```python
from build123d import *

# Parameters (mm, degrees)
SKETCH1_R           = 3.175
SKETCH1_R_2         = 2.286
BOSS_EXTRUDE1_DEPTH = 2.54
SKETCH2_R           = 3.175
BOSS_EXTRUDE2_DEPTH = 3.175


with BuildPart() as part:
    # Sketch1 → Boss-Extrude1 (new body)
    with BuildSketch(Plane(origin=(0, 0, 0), x_dir=(1, 0, 0), z_dir=(0, 1, 0))):
        with BuildLine():
            Line((2.54, 0), (10.16, 0))
            ThreePointArc((10.16, 0), (11.956051224, 0.743948776), (12.7, 2.54))
            Line((12.7, 2.54), (12.7, 25.4))
            ThreePointArc((12.7, 25.4), (6.35, 31.75), (0, 25.4))
            Line((0, 25.4), (0, 2.54))
            ThreePointArc((0, 2.54), (0.743948776, 0.743948776), (2.54, 0))
        make_face()
        with Locations((6.35, 25.4)):
            Circle(SKETCH1_R, mode=Mode.SUBTRACT)
        with Locations((6.35, 6.35)):
            Circle(SKETCH1_R_2, mode=Mode.SUBTRACT)
    extrude(amount=BOSS_EXTRUDE1_DEPTH)

    # Sketch2 → Boss-Extrude2 (add)
    with BuildSketch(Plane(origin=(0, 2.54, 0), x_dir=(1, 0, 0), z_dir=(0, 1, 0))):
        with BuildLine():
            Line((0, 25.4), (0, 16.256))
            Line((0, 16.256), (12.7, 16.256))
            Line((12.7, 16.256), (12.7, 25.4))
            ThreePointArc((12.7, 25.4), (6.35, 31.75), (0, 25.4))
        make_face()
        with Locations((6.35, 25.4)):
            Circle(SKETCH2_R, mode=Mode.SUBTRACT)
    extrude(amount=BOSS_EXTRUDE2_DEPTH)


solid = part.part
```
Could you check a few things on this model? Use its own coordinates, in mm. A direction names the side the tool comes from. Give positions to 0.01 mm unless a question says otherwise; leave off trailing zeros. Write each loop counter-clockwise with the first axis right and the second up, starting at its lowest first coordinate (ties: lowest second). Pieces come first, ordered by that corner, then holes. Notation, with made-up numbers: (48.25, 44.25) -> (84.25, 44.25) arc R26 cw to (84.25, 72.25) -> close; hole circle Ø6 at (28.5, 73). An arc over 180 degrees is marked (long way). Write each question's results on one line, items separated by ' | '.
1. Will these pins go through, and if not, where does the flat tip stop? pin 1 Ø1 at (x, z) = (9, -9) entering from +Y; pin 2 Ø3 at (x, y) = (10.5, 3) entering from -Z; pin 3 Ø2 at (y, z) = (4.5, -9.5) entering from +X; pin 4 Ø1.6 at (x, y) = (5.5, 3.5) entering from +Z.
Check sheet entries:
pin 1: stops at y = 2.54 | pin 2: stops at z = -31.17 | pin 3: passes through | pin 4: stops at z = -16.26
2. On a 3-axis mill with a long thin cutter (end or side, diameter ignored), from which of +Z, -Z, +X, -X, +Y, -Y can I reach the whole of each face in a straight line? I mean faces 4 (the flat face through (0, 2, -17)), 5 (the flat face through (6, 2.54, -10)). Say none if no direction works.
Check sheet entries:
face 4: +Z, -Z, -X, +Y, -Y | face 5: +Z, +X, -X, +Y
3. If we mould it in two halves opening along X, with no side actions, what happens to faces 1 (the cylindrical face through (5.94, 2.82, -28.55)), 2 (the flat face through (6, 4, -16.256)), 3 (the flat face through (12.7, 2, -16))? For each: released by +X, released by -X, zero draft, split by the parting line, or undercut.
Check sheet entries:
face 1: undercut | face 2: zero draft | face 3: released by +X
4. I want a section at A-A, the plane x = 6.35. Write out the boundary of the cut face in (y, z) (3 decimals), then the cut area to 3 significant figures.
Check sheet entries:
outline: (0, -31.75) -> (5.715, -31.75) -> (5.715, -28.575) -> (0, -28.575) -> close; (0, -22.225) -> (5.715, -22.225) -> (5.715, -16.256) -> (2.54, -16.256) -> (2.54, -8.636) -> (0, -8.636) -> close; (0, -4.064) -> (2.54, -4.064) -> (2.54, 0) -> (0, 0) -> close | area: 81.9 mm²
5. I want a section at B-B, the plane z = -26.5. Write out the boundary of the cut face in (x, y) (3 decimals), then the cut area to 3 significant figures.
Check sheet entries:
outline: (0.096, 0) -> (3.372, 0) -> (3.372, 5.715) -> (0.096, 5.715) -> close; (9.328, 0) -> (12.604, 0) -> (12.604, 5.715) -> (9.328, 5.715) -> close | area: 37.4 mm²
6. I want a section at D-D, the plane y = 4.65. Write out the boundary of the cut face in (x, z) (3 decimals).
Check sheet entries:
outline: (0, -25.4) arc R6.35 ccw to (12.7, -25.4) -> (12.7, -16.256) -> (0, -16.256) -> close; hole circle Ø6.35 at (6.35, -25.4)
7. I need wall thicknesses on L1, parallel to Z at x = 6.35, y = 1.25 (3 decimals); L2, parallel to X at y = 3.1, z = -25.4 (3 decimals); L3, parallel to Z at x = 5, y = 1.85. Which ranges of each line are inside material? Lowest first, please.
Check sheet entries:
L1: z = -31.75 to -28.575, -22.225 to -8.636, -4.064 to 0 | L2: x = 0 to 3.175, 9.525 to 12.7 | L3: z = -31.6 to -28.27, -22.53 to -8.19, -4.51 to 0
8. I want a section at C-C, the plane y = 1.1. Write out the boundary of the cut face in (x, z) (3 decimals), then the cut area to 3 significant figures.
Check sheet entries:
outline: (0, -25.4) arc R6.35 ccw to (12.7, -25.4) -> (12.7, -2.54) arc R2.54 ccw to (10.16, 0) -> (2.54, 0) arc R2.54 ccw to (0, -2.54) -> close; hole circle Ø6.35 at (6.35, -25.4); hole circle Ø4.572 at (6.35, -6.35) | area: 335 mm²
